For this review, take the finished solid that the model builds, in its own axes (mm). Face numbers are marked on the shaded views. A direction names the side the tool comes from. Give positions to 0.01 mm unless a question says otherwise; leave off trailing zeros. Order: outer loops, then holes, each group sorted by start corner. A loop starts at its lowest first (then second) coordinate and runs counter-clockwise, first axis right, second up.
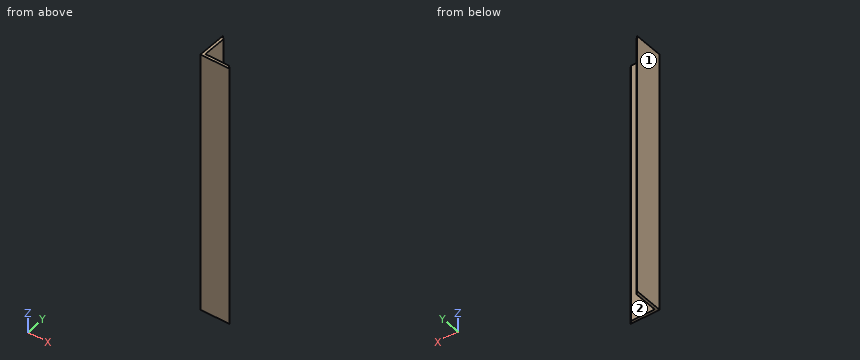
from build123d import *

# Parameters (mm, degrees)
BOSS_EXTRUDE1_DEPTH = 945
CUT_EXTRUDE1_DEPTH  = 956.523416772


with BuildPart() as part:
    # Sketch1 → Boss-Extrude1 (new body)
    with BuildSketch(Plane.XY):
        Polygon((-5, 100), (-5, -5), (100, -5), (100, 5), (5, 5), (5, 100), align=None)
    extrude(amount=BOSS_EXTRUDE1_DEPTH)

    # Sketch2 → Cut-Extrude1 (cut, through all)
    with BuildSketch(Plane.XY.offset(945)):
        Polygon((-5, 100), (100, -5), (100, 5), (5, 100), align=None)
    extrude(amount=-CUT_EXTRUDE1_DEPTH, mode=Mode.SUBTRACT)


solid = part.part
1) We need section A-A on y = 42.5. Give the boundary of the cut face in (x, z), then the cut area to 3 significant figures.
Answer sheet:
outline: (-5, 0) - (5, 0) - (5, 945) - (-5, 945) - close
area: 9,450 mm2
2) Tool access review of the marked faces 1 and 2: name each direction out of +Z, -Z, +X, -X, +Y, -Y from which nothing blocks a thin tool from reaching the whole face with its end or side.
Answer sheet:
face 1: +Z, -Z, -X, +Y, -Y
face 2: +Z, -Z, +X, +Y
3) We need section B-B on z = 242. Give the boundary of the cut face in (x, y), then the cut area to 3 significant figures.
Answer sheet:
outline: (-5, -5) - (100, -5) - (90, 5) - (5, 5) - (5, 90) - (-5, 100) - close
area: 1,900 mm2
4) Clearance check with a flat-ended pin moving along its axis: pin 1 (1.5 mm diameter, centred on y = 37.5, z = 746.5, fed in from +X). State where the tip first meets the part, or that it passes through.
Answer sheet:
pin 1: stops at x = 5
5) To check wall thickness, follow line 1 (Y direction, x = 21.5, z = 283.5); line 2 (Y direction, x = 92, z = 757). State the ranges of each line that lie inside material, in increasing order.
Answer sheet:
line 1: y = -5 to 5
line 2: y = -5 to 3
